```python
from build123d import *

# Parameters (mm, degrees)
F0_R     = 20.25
F0_R_2   = 17.75
F1_DEPTH = 45
F0_R_3   = 23.8
F2_DEPTH = 30
F3_R     = 21.3
F4_DEPTH = 24
F5_R     = 2


with BuildPart() as f1:
    # F0 (on Top) → F1 (new body)
    with BuildSketch(Plane.XY):
        Circle(F0_R)
        Circle(F0_R_2, mode=Mode.SUBTRACT)
    extrude(amount=F1_DEPTH)

    # F0 (on Top) → F2 (join)
    with BuildSketch(Plane.XY):
        Circle(F0_R_3)
        Circle(F0_R, mode=Mode.SUBTRACT)
    extrude(amount=F2_DEPTH)

    # F3 (on Top) → F4 (cut)
    with BuildSketch(Plane.XY):
        Circle(F3_R)
    extrude(amount=F4_DEPTH, mode=Mode.SUBTRACT)

    # F5
    f5_edges = [f1.edges().sort_by_distance(p)[0] for p in [
        (-17.75, 0, 24),
        (-21.3, 0, 0),
        (-17.75, 0, 45),
    ]]
    fillet(f5_edges, radius=F5_R)


solid = f1.part
```
Model file for the job. Use its own axes, mm. A direction names the side the tool comes from. Give positions to 0.01 mm unless a question says otherwise; leave off trailing zeros. Loops run counter-clockwise (first coordinate to the right, second up) from the corner with the lowest first, then second, coordinate; pieces in that order, holes last. Notation, with made-up numbers: (28, -40) - (57, -40) arc R16 ccw to (57, -15) - close; hole circle Ø6 at (21.25, 46.5). An arc over 180 degrees is marked (long way). One line per item, written item: value. Start each with the question number.
1. Which spindle directions (+Z, -Z, +X, -X, +Y, -Y) get a long thin tool onto all of the face, cutting with end or side? Do faces 1 (the flat face through (6, -19, 24)), 2 (the flat face through (4.41, -19.41, 45)). Say none if no direction does.
2. Pull direction X, two halves, no side cores. Call faces 3 (the flat face through (7, 20, 30)), 4 (the cylindrical face through (-3.848, -17.328, 34.381)), 5 (the cylindrical face through (11, 17, 37)): pulls with the +X half, pulls with the -X half, needs draft (parallel to the pull), parting line crosses it, or undercut.
3. Pin check, flat tips, straight feed: pin 1 (3 mm diameter, centred on x = 4, z = 35, fed in from +Y); pin 2 (1 mm diameter, centred on x = -11, z = 28, fed in from -Y); pin 3 (12 mm diameter, centred on x = 17.5, z = 32, fed in from -Y). Stop position of each tip, or through.
4. Probe L1, parallel to Y at x = 0, z = 14; L2, parallel to X at y = -11, z = 11.5; L3, parallel to X at y = -4.5, z = 8.5. List the from-to ranges inside material, lowest first. Write a range as from..to.
5. Slice it at A-A (x = 0). List the corners of the cut face in (y, z).
6. Slice it at D-D (z = 31). List the corners of the cut face in (x, y), plus the area to 3 significant figures.
7. Slice it at C-C (z = 15.5). List the corners of the cut face in (x, y), plus the area to 3 significant figures.
Solution:
1. face 1: -Z
1. face 2: +Z, +X, -X, +Y, -Y
2. face 3: needs draft
2. face 4: undercut
2. face 5: parting line crosses it
3. pin 1: stops at y = 20.1
3. pin 2: stops at y = -21.36
3. pin 3: stops at y = -20.64
4. L1: y = -23.8..-21.3, 21.3..23.8
4. L2: x = -21.11..-18.24, 18.24..21.11
4. L3: x = -23.37..-20.82, 20.82..23.37
5. outline: (-23.8, 0) - (-23.3, 0) arc R2 ccw to (-21.3, 2) - (-21.3, 24) - (-19.75, 24) arc R2 ccw to (-17.75, 26) - (-17.75, 43) arc R2 ccw to (-19.75, 45) - (-20.25, 45) - (-20.25, 30) - (-23.8, 30) - close; (17.75, 26) arc R2 ccw to (19.75, 24) - (21.3, 24) - (21.3, 2) arc R2 ccw to (23.3, 0) - (23.8, 0) - (23.8, 30) - (20.25, 30) - (20.25, 45) - (19.75, 45) arc R2 ccw to (17.75, 43) - close
6. outline: circle Ø40.5 at (0, 0); hole circle Ø35.5 at (0, 0)
6. area: 298 mm^2
7. outline: circle Ø47.6 at (0, 0); hole circle Ø42.6 at (0, 0)
7. area: 354 mm^2
